from build123d import *

# Parameters (mm, degrees)
SKETCH1_W           = 25
SKETCH1_H           = 40
BOSS_EXTRUDE1_DEPTH = 4.5
FILLET1_R           = 5
FILLET2_R           = 0.75


with BuildPart() as part:
    # Sketch1 → Boss-Extrude1 (new body)
    with BuildSketch(Plane.XY):
        with Locations((12.5, 20)):
            Rectangle(SKETCH1_W, SKETCH1_H)
        with BuildLine():
            Line((17.5, 30), (17.5, 10))
            ThreePointArc((17.5, 10), (12.5, 5), (7.5, 10))
            Line((7.5, 10), (7.5, 30))
            ThreePointArc((7.5, 30), (12.5, 35), (17.5, 30))
        make_face(mode=Mode.SUBTRACT)
    extrude(amount=BOSS_EXTRUDE1_DEPTH)

    # Fillet1
    fillet1_edges = [part.edges().sort_by_distance(p)[0] for p in [
        (0, 40, 2.25),
        (25, 40, 2.25),
        (25, 0, 2.25),
        (0, 0, 2.25),
    ]]
    fillet(fillet1_edges, radius=FILLET1_R)

    # Fillet2
    fillet2_edges = [part.edges().sort_by_distance(p)[0] for p in [
        (12.5, 35, 4.5),
        (7.5, 20, 4.5),
        (12.5, 5, 4.5),
        (17.5, 20, 4.5),
        (12.5, 40, 4.5),
        (25, 20, 4.5),
        (0, 20, 4.5),
        (12.5, 0, 4.5),
        (1.464466094, 38.535533906, 4.5),
        (1.464466094, 1.464466094, 4.5),
        (23.535533906, 1.464466094, 4.5),
        (23.535533906, 38.535533906, 4.5),
    ]]
    fillet(fillet2_edges, radius=FILLET2_R)


solid = part.part
Model file for the job. Use its own axes, mm. A direction names the side the tool comes from. Round coordinates to 2 decimals unless told otherwise and drop trailing zeros. Order: outer loops, then holes, each group sorted by start corner. A loop starts at its lowest first (then second) coordinate and runs counter-clockwise, first axis right, second up.
(1) Band-saw the part on A-A (x = 12.5). List the corners of the cut face in (y, z).
(2) Pull direction Y, two halves, no side cores. Call faces 1 (the face through (17.5, 20, 2)), 2 (the face through (23, 1, 2)), 3 (the face through (0, 20, 2)): released by +Y, released by -Y, zero draft, split by the parting line, or undercut.
(3) Drill centre lines: line 1 (X direction, y = 23, z = 3.35); line 2 (Y direction, x = 14.25, z = 2.3); line 3 (Y direction, x = 10.25, z = 3.8). Where is each one in solid material? Low to high.
(4) 3-axis set-ups, long thin cutter, end or side, ignore diameter. For faces 4 (the face through (25, 20, 2)), 5 (the face through (7.5, 20, 2)): which of +Z, -Z, +X, -X, +Y, -Y reach the whole face in a straight line?
(5) Band-saw the part on B-B (y = 16.5). List the corners of the cut face in (x, z), then the cut area to 3 significant figures.
(6) Band-saw the part on C-C (z = 1.1). List the corners of the cut face in (x, y).
Verdict:
1. outline: (0, 0) - (5, 0) - (5, 3.75) arc R0.75 ccw to (4.25, 4.5) - (0.75, 4.5) arc R0.75 ccw to (0, 3.75) - close; (35, 0) - (40, 0) - (40, 3.75) arc R0.75 ccw to (39.25, 4.5) - (35.75, 4.5) arc R0.75 ccw to (35, 3.75) - close
2. face 1: undercut
2. face 2: released by -Y
2. face 3: zero draft
3. line 1: x = 0 to 7.5, 17.5 to 25
3. line 2: y = 0 to 5.32, 34.68 to 40
3. line 3: y = 0 to 5.53, 34.47 to 40
4. face 4: +Z, -Z, +X, +Y, -Y
4. face 5: +Z, -Z
5. outline: (0, 0) - (7.5, 0) - (7.5, 3.75) arc R0.75 ccw to (6.75, 4.5) - (0.75, 4.5) arc R0.75 ccw to (0, 3.75) - close; (17.5, 0) - (25, 0) - (25, 3.75) arc R0.75 ccw to (24.25, 4.5) - (18.25, 4.5) arc R0.75 ccw to (17.5, 3.75) - close
5. area: 67.0 mm2
6. outline: (0, 5) arc R5 ccw to (5, 0) - (20, 0) arc R5 ccw to (25, 5) - (25, 35) arc R5 ccw to (20, 40) - (5, 40) arc R5 ccw to (0, 35) - close; hole (7.5, 10) arc R5 ccw to (17.5, 10) - (17.5, 30) arc R5 ccw to (7.5, 30) - close
